Could you check a few things on this model? Use its own coordinates, in mm. A direction names the side the tool comes from. Give positions to 0.01 mm unless a question says otherwise; leave off trailing zeros. Loops run counter-clockwise (first coordinate to the right, second up) from the corner with the lowest first, then second, coordinate; pieces in that order, holes last. Notation, with made-up numbers: (81, 30.5) - (127, 30.5) arc R16 cw to (127, 35.5) - close; hole circle Ø5 at (-37.75, -31). An arc over 180 degrees is marked (long way). One line per item, written item: value. Start each with the question number.
Q1. If we mould it in two halves opening along Z, with no side actions, what happens to faces 1 (the face through (12, 1, -84)), 2 (the face through (17, 6, -8)), 3 (the face through (4, -13, -77))? For each: released by +Z, released by -Z, zero draft, split by the parting line, or undercut.
Q2. I want a section at D-D (z = -41.5). Please give me the cut outline in (x, y), then the cut area to 3 significant figures.
Q3. I'm going to push flat-ended pins straight in: P1, Ø1, axis at x = -1, z = -47.5, coming from the +Y side; P2, Ø2, axis at y = 3, z = -8.5, coming from the +X side; P3, Ø3, axis at y = 3.5, z = -51.5, coming from the +X side; P4, Ø1.2, axis at x = 3.5, z = -77.1, coming from the -Y side. Where does each tip first touch, or does it pass through?
Q4. I want a section at C-C (x = 22.5). Please give me the cut outline in (y, z), then the cut area to 3 significant figures.
Q5. I want a section at A-A (z = -8). Please give me the cut outline in (x, y).
Q6. I want a section at B-B (x = 7.75). Please give me the cut outline in (y, z), then the cut area to 3 significant figures.
Q7. For faces 4 (the face through (16.117, -18.07, -57.976)), 5 (the face through (-3, 6, -68)), 6 (the face through (19, 4.302, -68)), which set-ups out of +Z, -Z, +X, -X, +Y, -Y let a thin tool reach every point of the face, with its end or its side?
Q8. If I drill on line 1 (Z direction, x = 12.5, y = -3); line 2 (Z direction, x = 12.25, y = 1); line 3 (X direction, y = -19.75, z = -17.1), over which ranges is the centre line in solid material (lowest first)? Write a range as from..to.
```python
from build123d import *

# Parameters (mm, degrees)
SKETCH1_W           = 25
SKETCH1_H           = 46
SKETCH1_W_2         = 2.5
SKETCH1_H_2         = 12.2
BOSS_EXTRUDE1_DEPTH = 3
R_VOLUTION1_START   = -4.25
R_VOLUTION1_DEPTH   = 6.75
R_VOLUTION1_START_2 = 0.5
R_VOLUTION1_2_DEPTH = 2
R_VOLUTION1_3_DEPTH = 2
SKETCH9_W           = 11.354173072
SKETCH9_H           = 3.73743218
SKETCH9_W_2         = 2
SKETCH9_H_2         = 6
CUT_EXTRUDE2_DEPTH  = 6
CUT_EXTRUDE8_DEPTH  = 0.5
BOSS_EXTRUDE2_DEPTH = 23
SKETCH10_R          = 1
CUT_EXTRUDE3_DEPTH  = 10
SKETCH11_W          = 15
SKETCH11_H          = 9
BOSS_EXTRUDE3_DEPTH = 3
SKETCH12_W          = 5
SKETCH12_H          = 4.302239334
CUT_EXTRUDE4_DEPTH  = 13
SKETCH1_10_W        = 1
SKETCH1_10_H        = 5
BOSS_EXTRUDE4_DEPTH = 18
CUT_EXTRUDE5_DEPTH  = 1
CUT_EXTRUDE9_DEPTH  = 0.5


with BuildPart() as part:
    # Sketch1 → Boss-Extrude1 (new body)
    with BuildSketch(Plane(origin=(0, 0, 0), x_dir=(1, 0, 0), z_dir=(0, 1, 0))):
        with Locations((12.5, 15)):
            Rectangle(SKETCH1_W, SKETCH1_H)
        with Locations((5.4, 8)):
            Rectangle(SKETCH1_W_2, SKETCH1_H_2, mode=Mode.SUBTRACT)
    boss_extrude1 = extrude(amount=BOSS_EXTRUDE1_DEPTH)

    # Révolution1: read off the stored shape, not the designer's step
    # Révolution1 outline → Révolution1 (add)
    with BuildSketch(Plane.YZ.offset(R_VOLUTION1_START)):
        with BuildLine():
            Line((-6, 9), (-6, 7))
            ThreePointArc((-6, 7), (9, -8), (-6, -23))
            Line((-6, -23), (-6, -25))
            ThreePointArc((-6, -25), (11, -8), (-6, 9))
        make_face()
    r_volution1 = extrude(amount=R_VOLUTION1_DEPTH)

    # R_volution1 2 outline → R_volution1 2 (add)
    with BuildSketch(Plane.YZ.offset(R_VOLUTION1_START_2)):
        with BuildLine():
            ThreePointArc((-6, 1), (-2.788601192, 0.407551231), (0, -1.291796068))
            Line((0, -1.291796068), (0, 5.747727085))
            ThreePointArc((0, 5.747727085), (-2.935355345, 6.683594694), (-6, 7))
            Line((-6, 7), (-6, 1))
        make_face()
        with BuildLine():
            ThreePointArc((0, -14.708203932), (-2.788601192, -16.407551231), (-6, -17))
            Line((-6, -17), (-6, -23))
            ThreePointArc((-6, -23), (-2.935355345, -22.683594694), (0, -21.747727085))
            Line((0, -21.747727085), (0, -14.708203932))
        make_face()
        with BuildLine():
            Line((3, 4), (3, -20))
            ThreePointArc((3, -20), (9, -8), (3, 4))
        make_face()
    r_volution1_2 = extrude(amount=R_VOLUTION1_2_DEPTH)

    # R_volution1 3 outline → R_volution1 3 (add)
    with BuildSketch(Plane.YZ.offset(R_VOLUTION1_START)):
        with BuildLine():
            Line((-6, 7), (-6, 4))
            ThreePointArc((-6, 4), (6, -8), (-6, -20))
            Line((-6, -20), (-6, -23))
            ThreePointArc((-6, -23), (9, -8), (-6, 7))
        make_face()
    r_volution1_3 = extrude(amount=R_VOLUTION1_3_DEPTH)

    # Sketch9 → Cut-Extrude2 (cut)
    with BuildSketch(Plane(origin=(0, -6, 0), x_dir=(-1, 0, 0), z_dir=(0, -1, 0))):
        with Locations((-5.677086536, 24.86871609)):
            Rectangle(SKETCH9_W, SKETCH9_H)
        Polygon((0, -9), (0, -7), (-0.5, -7), (-2.5, -7), (-2.5, -9), align=None)
        Polygon((0, -9.458628642), (0, -9), (-2.5, -9), (-2.5, -7), (-11.354173072, -7), (-11.354173072, -9.458628642), align=None)
        with Locations((-1.5, -4)):
            Rectangle(SKETCH9_W_2, SKETCH9_H_2)
        Polygon((0, -7), (2.25, -7), (2.25, -4), (2.25, 23), (0, 23), (-11.354173072, 23), (-11.354173072, -7), (-2.5, -7), (-2.5, -1), (-0.5, -1), (-0.5, -7), align=None)
    extrude(amount=-CUT_EXTRUDE2_DEPTH, mode=Mode.SUBTRACT)

    # Cut-Extrude8: read off the stored shape, not the designer's step
    # Cut-Extrude8 outline → Cut-Extrude8 (cut)
    with BuildSketch(Plane.YZ):
        with BuildLine():
            Line((0, 5.747727085), (0, -21.747727085))
            ThreePointArc((0, -21.747727085), (1.550737546, -20.960955309), (3, -20))
            Line((3, -20), (3, 4))
            ThreePointArc((3, 4), (1.550737546, 4.960955309), (0, 5.747727085))
        make_face()
    extrude(amount=CUT_EXTRUDE8_DEPTH, mode=Mode.SUBTRACT)

    # Sketch1<9> → Boss-Extrude2 (add)
    with BuildSketch(Plane(origin=(0, 0, 0), x_dir=(1, 0, 0), z_dir=(0, 1, 0))):
        with BuildLine():
            ThreePointArc((5.177050983, 17.6), (1.75, 17.1), (5.177050983, 16.6))
            Line((5.177050983, 16.6), (5.177050983, 17.6))
        make_face()
        with BuildLine():
            Line((5.177050983, -1.6), (5.177050983, -0.6))
            ThreePointArc((5.177050983, -0.6), (1.75, -1.1), (5.177050983, -1.6))
        make_face()
        with BuildLine():
            ThreePointArc((14.822949017, 16.6), (18.25, 17.1), (14.822949017, 17.6))
            Line((14.822949017, 17.6), (14.822949017, 16.6))
        make_face()
        with BuildLine():
            Line((14.822949017, -0.6), (14.822949017, -1.6))
            ThreePointArc((14.822949017, -1.6), (18.25, -1.1), (14.822949017, -0.6))
        make_face()
    boss_extrude2 = extrude(amount=-BOSS_EXTRUDE2_DEPTH)

    # Sketch10 → Cut-Extrude3 (cut)
    with BuildSketch(Plane(origin=(0, -23, 0), x_dir=(-1, 0, 0), z_dir=(0, -1, 0))):
        with Locations(Location((-3.5, -1.1, 0), (0, 0, 90))):
            Circle(SKETCH10_R)
        with Locations(Location((-16.5, -1.1, 0), (0, 0, 90))):
            Circle(SKETCH10_R)
        with Locations(Location((-16.5, 17.1, 0), (0, 0, 90))):
            Circle(SKETCH10_R)
        with Locations(Location((-3.5, 17.1, 0), (0, 0, 90))):
            Circle(SKETCH10_R)
    cut_extrude3 = extrude(amount=-CUT_EXTRUDE3_DEPTH, mode=Mode.SUBTRACT)

    # Sketch11 → Boss-Extrude3 (add)
    with BuildSketch(Plane(origin=(0, 3, 0), x_dir=(1, 0, 0), z_dir=(0, 1, 0))):
        with Locations((17.5, 8)):
            Rectangle(SKETCH11_W, SKETCH11_H)
    boss_extrude3 = extrude(amount=BOSS_EXTRUDE3_DEPTH)

    # Sketch12 → Cut-Extrude4 (cut)
    with BuildSketch(Plane(origin=(25, 0, 0), x_dir=(0, 0, -1), z_dir=(1, 0, 0))):
        with Locations((8, 2.151119667)):
            Rectangle(SKETCH12_W, SKETCH12_H)
    cut_extrude4 = extrude(amount=-CUT_EXTRUDE4_DEPTH, mode=Mode.SUBTRACT)

    # Sketch1<10> → Boss-Extrude4 (add)
    with BuildSketch(Plane(origin=(0, 0, 0), x_dir=(1, 0, 0), z_dir=(0, 1, 0))):
        with BuildLine():
            Line((14.822949017, -1.6), (14.822949017, -0.6))
            ThreePointArc((14.822949017, -0.6), (14.75, -1.1), (14.822949017, -1.6))
        make_face()
        with BuildLine():
            Line((14.822949017, -0.6), (13.541960108, -0.6))
            ThreePointArc((13.541960108, -0.6), (13.5, -1.1), (13.541960108, -1.6))
            Line((13.541960108, -1.6), (14.822949017, -1.6))
            ThreePointArc((14.822949017, -1.6), (14.75, -1.1), (14.822949017, -0.6))
        make_face()
        with BuildLine():
            ThreePointArc((6.5, -1.1), (6.489491568, -1.350878781), (6.458039892, -1.6))
            Line((6.458039892, -1.6), (9.5, -1.6))
            Line((9.5, -1.6), (10.5, -1.6))
            Line((10.5, -1.6), (13.541960108, -1.6))
            ThreePointArc((13.541960108, -1.6), (13.5, -1.1), (13.541960108, -0.6))
            Line((13.541960108, -0.6), (6.458039892, -0.6))
            ThreePointArc((6.458039892, -0.6), (6.489491568, -0.849121219), (6.5, -1.1))
        make_face()
        with Locations((10, -4.1)):
            Rectangle(SKETCH1_10_W, SKETCH1_10_H)
        with BuildLine():
            Line((5.177050983, -1.6), (6.458039892, -1.6))
            ThreePointArc((6.458039892, -1.6), (6.489491568, -1.350878781), (6.5, -1.1))
            ThreePointArc((6.5, -1.1), (6.489491568, -0.849121219), (6.458039892, -0.6))
            Line((6.458039892, -0.6), (5.177050983, -0.6))
            ThreePointArc((5.177050983, -0.6), (5.231666715, -0.847353231), (5.25, -1.1))
            ThreePointArc((5.25, -1.1), (5.231666715, -1.352646769), (5.177050983, -1.6))
        make_face()
        with BuildLine():
            Line((5.177050983, -0.6), (5.177050983, -1.6))
            ThreePointArc((5.177050983, -1.6), (5.231666715, -1.352646769), (5.25, -1.1))
            ThreePointArc((5.25, -1.1), (5.231666715, -0.847353231), (5.177050983, -0.6))
        make_face()
        with BuildLine():
            ThreePointArc((13.541960108, 17.6), (13.5, 17.1), (13.541960108, 16.6))
            Line((13.541960108, 16.6), (14.822949017, 16.6))
            ThreePointArc((14.822949017, 16.6), (14.75, 17.1), (14.822949017, 17.6))
            Line((14.822949017, 17.6), (13.541960108, 17.6))
        make_face()
        with BuildLine():
            ThreePointArc((14.822949017, 17.6), (14.75, 17.1), (14.822949017, 16.6))
            Line((14.822949017, 16.6), (14.822949017, 17.6))
        make_face()
        with BuildLine():
            Line((9.5, 17.6), (6.458039892, 17.6))
            ThreePointArc((6.458039892, 17.6), (6.489491568, 17.350878781), (6.5, 17.1))
            ThreePointArc((6.5, 17.1), (6.489491568, 16.849121219), (6.458039892, 16.6))
            Line((6.458039892, 16.6), (13.541960108, 16.6))
            ThreePointArc((13.541960108, 16.6), (13.5, 17.1), (13.541960108, 17.6))
            Line((13.541960108, 17.6), (10.5, 17.6))
            Line((10.5, 17.6), (9.5, 17.6))
        make_face()
        with BuildLine():
            ThreePointArc((6.5, 17.1), (6.489491568, 17.350878781), (6.458039892, 17.6))
            Line((6.458039892, 17.6), (5.177050983, 17.6))
            ThreePointArc((5.177050983, 17.6), (5.231666715, 17.352646769), (5.25, 17.1))
            ThreePointArc((5.25, 17.1), (5.231666715, 16.847353231), (5.177050983, 16.6))
            Line((5.177050983, 16.6), (6.458039892, 16.6))
            ThreePointArc((6.458039892, 16.6), (6.489491568, 16.849121219), (6.5, 17.1))
        make_face()
        with BuildLine():
            ThreePointArc((5.25, 17.1), (5.231666715, 17.352646769), (5.177050983, 17.6))
            Line((5.177050983, 17.6), (5.177050983, 16.6))
            ThreePointArc((5.177050983, 16.6), (5.231666715, 16.847353231), (5.25, 17.1))
        make_face()
        with Locations((10, 20.1)):
            Rectangle(SKETCH1_10_W, SKETCH1_10_H)
    boss_extrude4 = extrude(amount=-BOSS_EXTRUDE4_DEPTH)

    # Sketch14 → Cut-Extrude5 (cut)
    with BuildSketch(Plane.ZY.offset(-9.5)):
        Polygon((-22.6, 0), (-17.6, -18), (-22.6, -18), align=None)
        Polygon((6.6, -18), (6.6, 0), (1.6, -18), align=None)
    cut_extrude5 = extrude(amount=-CUT_EXTRUDE5_DEPTH, mode=Mode.SUBTRACT)

    # Mirror2: Boss-Extrude1, Révolution1, R_volution1 2, R_volution1 3, Boss-Extrude2, Cut-Extrude3, Boss-Extrude3, Cut-Extrude4, Boss-Extrude4, Cut-Extrude5 across plane
    add(boss_extrude1.mirror(Plane(origin=(0, 3, -38), x_dir=(1, 0, 0), z_dir=(0, 0, -1))))
    add(r_volution1.mirror(Plane(origin=(0, 3, -38), x_dir=(1, 0, 0), z_dir=(0, 0, -1))))
    add(r_volution1_2.mirror(Plane(origin=(0, 3, -38), x_dir=(1, 0, 0), z_dir=(0, 0, -1))))
    add(r_volution1_3.mirror(Plane(origin=(0, 3, -38), x_dir=(1, 0, 0), z_dir=(0, 0, -1))))
    add(boss_extrude2.mirror(Plane(origin=(0, 3, -38), x_dir=(1, 0, 0), z_dir=(0, 0, -1))))
    add(cut_extrude3.mirror(Plane(origin=(0, 3, -38), x_dir=(1, 0, 0), z_dir=(0, 0, -1))), mode=Mode.SUBTRACT)
    add(boss_extrude3.mirror(Plane(origin=(0, 3, -38), x_dir=(1, 0, 0), z_dir=(0, 0, -1))))
    add(cut_extrude4.mirror(Plane(origin=(0, 3, -38), x_dir=(1, 0, 0), z_dir=(0, 0, -1))), mode=Mode.SUBTRACT)
    add(boss_extrude4.mirror(Plane(origin=(0, 3, -38), x_dir=(1, 0, 0), z_dir=(0, 0, -1))))
    add(cut_extrude5.mirror(Plane(origin=(0, 3, -38), x_dir=(1, 0, 0), z_dir=(0, 0, -1))), mode=Mode.SUBTRACT)

    # Cut-Extrude9: read off the stored shape, not the designer's step
    # Cut-Extrude9 outline → Cut-Extrude9 (cut)
    with BuildSketch(Plane.YZ):
        with BuildLine():
            Line((0, -54.252272915), (0, -81.747727085))
            ThreePointArc((0, -81.747727085), (1.550737546, -80.960955309), (3, -80))
            Line((3, -80), (3, -56))
            ThreePointArc((3, -56), (1.550737546, -55.039044691), (0, -54.252272915))
        make_face()
    extrude(amount=CUT_EXTRUDE9_DEPTH, mode=Mode.SUBTRACT)


solid = part.part
```
Worked answers:
1. face 1: released by -Z
1. face 2: zero draft
1. face 3: undercut
2. outline: (0, 0) - (25, 0) - (25, 3) - (0, 3) - close
2. area: 75.0 mm²
3. P1: passes through
3. P2: stops at x = 12
3. P3: stops at x = 25
3. P4: stops at y = -13
4. outline: (0, -84) - (3, -84) - (3, -72.5) - (6, -72.5) - (6, -63.5) - (3, -63.5) - (3, -12.5) - (6, -12.5) - (6, -3.5) - (3, -3.5) - (3, 8) - (0, 8) - (0, -5.5) - (4.3, -5.5) - (4.3, -10.5) - (0, -10.5) - (0, -65.5) - (4.3, -65.5) - (4.3, -70.5) - (0, -70.5) - close
4. area: 287 mm²
5. outline: (-4.25, 6) - (-2.25, 6) - (-2.25, 9) - (0.5, 9) - (0.5, 0) - (4.15, 0) - (4.15, 3) - (2.5, 3) - (2.5, 11) - (-4.25, 11) - close; (6.65, 0) - (12, 0) - (12, 4.3) - (25, 4.3) - (25, 6) - (10, 6) - (10, 3) - (6.65, 3) - close
6. outline: (-18, -77.6) - (0, -77.6) - (0, -84) - (3, -84) - (3, 8) - (0, 8) - (0, 1.6) - (-18, 1.6) - (-18, 0.6) - (0, 0.6) - (0, -16.6) - (-18, -16.6) - (-18, -17.6) - (0, -17.6) - (0, -58.4) - (-18, -58.4) - (-18, -59.4) - (0, -59.4) - (0, -76.6) - (-18, -76.6) - close
6. area: 348 mm²
7. face 4: -Y
7. face 5: -X, -Y
7. face 6: +X, -Y
8. line 1: z = -77.6..-76.6, -59.4..-58.4, -17.6..-16.6, 0.6..1.6
8. line 2: z = -84..-70.5, -65.5..-10.5, -5.5..8
8. line 3: x = 1.75..2.5, 4.5..5.18, 14.82..15.5, 17.5..18.25
